Design review of the part shown in the three views and the two pictorial views. Dimensions are in mm from the part's minimum x, y and z. A direction names the side the tool comes from. Coordinates: 2 decimals unless noted, no trailing zeros. Order: outer loops, then holes, each group sorted by start corner. A loop starts at its lowest first (then second) coordinate and runs counter-clockwise, first axis right, second up. Notation, with made-up numbers: (29.5, -10.5) -> (39.5, -10.5) arc R28 cw to (39.5, 23.5) -> close; hole circle Ø3 at (1, 23). An arc over 180 degrees is marked (long way). Answer as a JSON object with one key per item and string values. Group by question number.
1) Machinability: for the marked faces 1 and 2, which of the approach directions +Z, -Z, +X, -X, +Y, -Y give a long, thin tool a straight path to every point of the face, cutting with its end or side? Answer none if there is none.
2) Add section B-B, the plane z = 6.5. Write out the cut boundary in (x, y), then the cut area to 3 significant figures.
3) Add section C-C, the plane y = 21. Write out the cut boundary in (x, z), then the cut area to 3 significant figures.
4) For pin 1 (1.3 mm diameter, centred on x = 1, z = 1.5, fed in from -Y); pin 2 (4 mm diameter, centred on x = 75.5, y = 37, fed in from +Z); pin 3 (2 mm diameter, centred on y = 50, z = 8.5, fed in from -X), all flat-tipped, find the tip position at first contact; note any pin that passes through.
5) Add section A-A, the plane y = 30.3. Write out the cut boundary in (x, z).
6) Wall thickness on L1, parallel to X at y = 56, z = 4; L2, parallel to Z at x = 5, y = 47: over which ranges is each line inside the solid? List them lowest first.
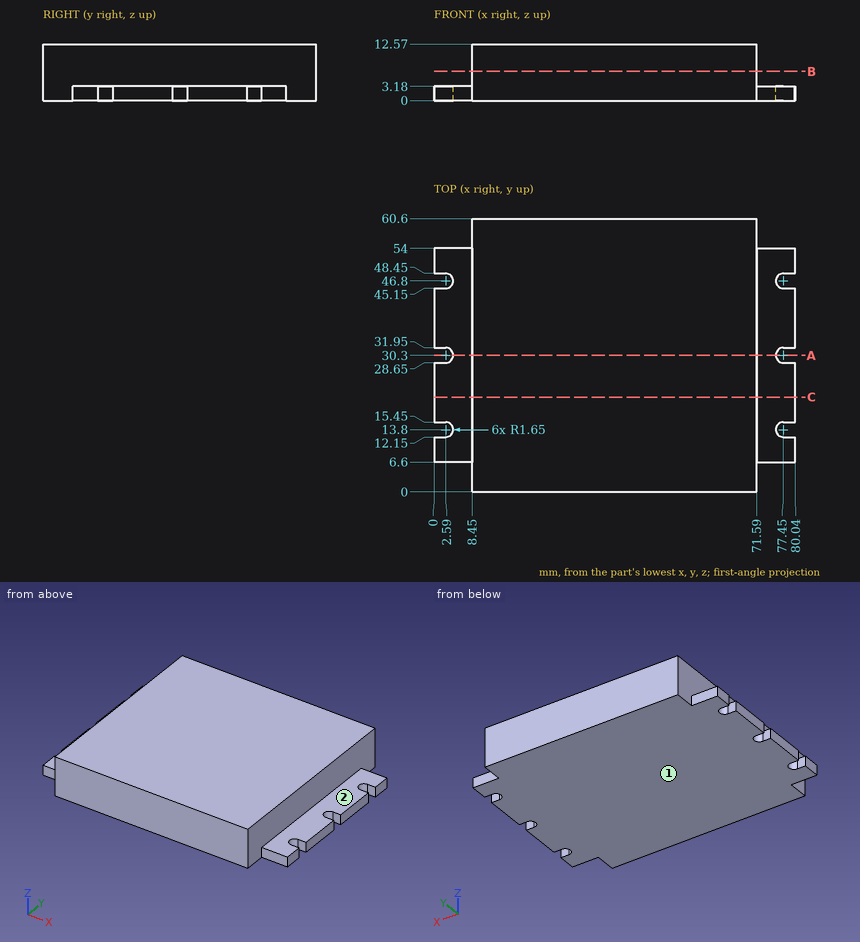
Output values:
{
 "1": {"face 1": "-Z, +X, -X, +Y, -Y", "face 2": "+Z, +X, +Y, -Y"},
 "2": {"outline": "(8.45, 0) -> (71.59, 0) -> (71.59, 60.6) -> (8.45, 60.6) -> close", "area": "3,830 mm²"},
 "3": {"outline": "(0, 0) -> (80.04, 0) -> (80.04, 3.18) -> (71.59, 3.18) -> (71.59, 12.57) -> (8.45, 12.57) -> (8.45, 3.18) -> (0, 3.18) -> close", "area": "847 mm²"},
 "4": {"pin 1": "stops at y = 6.6", "pin 2": "stops at z = 3.18", "pin 3": "stops at x = 8.45"},
 "5": {"outline": "(4.24, 0) -> (75.8, 0) -> (75.8, 3.18) -> (71.59, 3.18) -> (71.59, 12.57) -> (8.45, 12.57) -> (8.45, 3.18) -> (4.24, 3.18) -> close"},
 "6": {"L1": "x = 8.45 to 71.59", "L2": "z = 0 to 3.18"}
}
